from build123d import *

# Parameters (mm, degrees)
SKETCH1_R           = 62.5
SKETCH1_R_2         = 1.5
BOSS_EXTRUDE1_DEPTH = 2
SKETCH2_R           = 11.3
BOSS_EXTRUDE2_DEPTH = 5
SECTORS_DEPTH       = 89.529656048
SKETCH_1_R          = 10
CUT_EXTRUDE_1_DEPTH = 89.665100237
CHAMFER_1_SIZE      = 0.5


with BuildPart() as part:
    # Sketch1 → Boss-Extrude1 (new body)
    with BuildSketch(Plane.XY):
        Circle(SKETCH1_R)
        with Locations((-57.5, 0)):
            Circle(SKETCH1_R_2, mode=Mode.SUBTRACT)
        with Locations((0, 57.5)):
            Circle(SKETCH1_R_2, mode=Mode.SUBTRACT)
        with Locations((57.5, 0)):
            Circle(SKETCH1_R_2, mode=Mode.SUBTRACT)
        with Locations((0, -57.5)):
            Circle(SKETCH1_R_2, mode=Mode.SUBTRACT)
        with Locations((-15, 0)):
            Circle(SKETCH1_R_2, mode=Mode.SUBTRACT)
        with Locations(Location((15, 0, 0), (0, 0, 180))):
            Circle(SKETCH1_R_2, mode=Mode.SUBTRACT)
    extrude(amount=BOSS_EXTRUDE1_DEPTH)

    # Sketch2 → Boss-Extrude2 (add)
    with BuildSketch(Plane.XY.offset(2)):
        Circle(SKETCH2_R)
    extrude(amount=BOSS_EXTRUDE2_DEPTH)

    # Sector (Cut Extrude) → Sectors (cut, through all)
    with BuildSketch(Plane.XY.offset(2)):
        with BuildLine():
            Line((20.5742201, -5.512845661), (50.71110588, -13.587999868))
            ThreePointArc((50.71110588, -13.587999868), (37.123106012, -37.123106012), (13.587999868, -50.71110588))
            Line((13.587999868, -50.71110588), (5.512845661, -20.5742201))
            ThreePointArc((5.512845661, -20.5742201), (15.061374439, -15.061374439), (20.5742201, -5.512845661))
        make_face()
        with BuildLine():
            Line((-20.5742201, -5.512845661), (-50.71110588, -13.587999868))
            ThreePointArc((-50.71110588, -13.587999868), (-37.123106012, -37.123106012), (-13.587999868, -50.71110588))
            Line((-13.587999868, -50.71110588), (-5.512845661, -20.5742201))
            ThreePointArc((-5.512845661, -20.5742201), (-15.061374439, -15.061374439), (-20.5742201, -5.512845661))
        make_face()
        with BuildLine():
            Line((-5.512845661, 20.5742201), (-13.587999868, 50.71110588))
            ThreePointArc((-13.587999868, 50.71110588), (-37.123106012, 37.123106012), (-50.71110588, 13.587999868))
            Line((-50.71110588, 13.587999868), (-20.5742201, 5.512845661))
            ThreePointArc((-20.5742201, 5.512845661), (-15.061374439, 15.061374439), (-5.512845661, 20.5742201))
        make_face()
        with BuildLine():
            Line((20.5742201, 5.512845661), (50.71110588, 13.587999868))
            ThreePointArc((50.71110588, 13.587999868), (37.123106012, 37.123106012), (13.587999868, 50.71110588))
            Line((13.587999868, 50.71110588), (5.512845661, 20.5742201))
            ThreePointArc((5.512845661, 20.5742201), (15.061374439, 15.061374439), (20.5742201, 5.512845661))
        make_face()
    extrude(amount=-SECTORS_DEPTH, mode=Mode.SUBTRACT)

    # Эскиз1 → Вырез-Вытянуть1 (cut, through all)
    with BuildSketch(Plane.XY.offset(7)):
        Circle(SKETCH_1_R)
    extrude(amount=-CUT_EXTRUDE_1_DEPTH, mode=Mode.SUBTRACT)

    # Фаска1
    chamfer_1_edges = [part.edges().sort_by_distance(p)[0] for p in [
        (-11.3, 0, 7),
    ]]
    chamfer(chamfer_1_edges, length=CHAMFER_1_SIZE)


solid = part.part
Could you check a few things on this model? Use its own coordinates, in mm. Give positions to 0.01 mm unless a question says otherwise; leave off trailing zeros. Order: outer loops, then holes, each group sorted by start corner. A loop starts at its lowest first (then second) coordinate and runs counter-clockwise, first axis right, second up. Notation, with made-up numbers: (14, 53) -> (43, 53) arc R17 ccw to (43, 61) -> close; hole circle Ø1 at (38, -3). An arc over 180 degrees is marked (long way). Answer in a Markdown table with one row per item. Add a question column.
Item 1: Imagine slicing it at D-D (y = 0). Count the separate pieces of the cut face and the enclosed holes in it, and give its area (3 significant figures).
Item 2: I'm going to push flat-ended pins straight in: P1, Ø4, axis at x = 15, y = 0, coming from the +Z side; P2, Ø4, axis at x = -3.5, z = 2, coming from the +Y side; P3, Ø1, axis at x = 2.5, z = 1.5, coming from the -Y side. Where does each tip first touch, or does it pass through?
Item 3: Imagine slicing it at B-B (y = -22). List the corners of the cut face in (x, z) for me, and give its area (3 significant figures).
Item 4: Imagine slicing it at C-C (x = 38.5). List the corners of the cut face in (y, z) for me.
Item 5: Imagine slicing it at A-A (x = 0). List the corners of the cut face in (y, z) for me, and give its area (3 significant figures).
Item 6: Please list where these lines run through material, in increasing order: probe 1 along Y at (x, z) = (0, 0.55); probe 2 along Y at (x, z) = (14, 1.25); probe 3 along Z at (x, y) = (45, -40.5).
Item 7: We'd pull the mould along Y, two halves only. Please class faces 1 (the cylindrical face through (14.95, 15.17, 1.01)), 2 (the flat face through (13, 1, 0)), 3 (the cylindrical face through (-62.44, 2.75, 0.99)): pulls with the +Y half, pulls with the -Y half, needs draft (parallel to the pull), parting line crosses it, or undercut.
Result:
| question | item | result |
|---|---|---|
| 1 | separate pieces | 6 |
| 1 | enclosed holes | 0 |
| 1 | area | 199 mm2 |
| 2 | P1 | z = 2 |
| 2 | P2 | y = 62.48 |
| 2 | P3 | y = -62.47 |
| 3 | outline | (-58.5, 0) -> (-47.67, 0) -> (-47.67, 2) -> (-58.5, 2) -> close; (-5.89, 0) -> (5.89, 0) -> (5.89, 2) -> (-5.89, 2) -> close; (47.67, 0) -> (58.5, 0) -> (58.5, 2) -> (47.67, 2) -> close |
| 3 | area | 66.9 mm2 |
| 4 | outline | (-49.23, 0) -> (-35.69, 0) -> (-35.69, 2) -> (-49.23, 2) -> close; (-10.32, 0) -> (10.32, 0) -> (10.32, 2) -> (-10.32, 2) -> close; (35.69, 0) -> (49.23, 0) -> (49.23, 2) -> (35.69, 2) -> close |
| 5 | outline | (-62.5, 0) -> (-59, 0) -> (-59, 2) -> (-62.5, 2) -> close; (-56, 0) -> (-10, 0) -> (-10, 7) -> (-10.8, 7) -> (-11.3, 6.5) -> (-11.3, 2) -> (-56, 2) -> close; (10, 0) -> (56, 0) -> (56, 2) -> (11.3, 2) -> (11.3, 6.5) -> (10.8, 7) -> (10, 7) -> close; (59, 0) -> (62.5, 0) -> (62.5, 2) -> (59, 2) -> close |
| 5 | area | 211 mm2 |
| 6 | probe 1 | -62.5 to -59, -56 to -10, 10 to 56, 59 to 62.5 |
| 6 | probe 2 | -60.91 to -50.6, -16.05 to -1.12, 1.12 to 16.05, 50.6 to 60.91 |
| 6 | probe 3 | 0 to 2 |
| 7 | face 1 | undercut |
| 7 | face 2 | needs draft |
| 7 | face 3 | parting line crosses it |
